Geometry: see drawing. Coordinates: mm, zero at the bounding-box minimum. Coordinates: 2 decimals unless noted, no trailing zeros. Write each loop counter-clockwise with the first axis right and the second up, starting at its lowest first coordinate (ties: lowest second). Pieces come first, ordered by that corner, then holes.
1) Line query: L1, parallel to Y at x = 280, z = 3.4. Output: solid intervals per line, ascending.
2) Section query B-B (y = 10). State how many separate pieces and enclosed holes the cut face has, then the cut area to 4 significant figures.
3) Section query A-A (x = 20). Output: boundary loops of the cut face in (y, z).
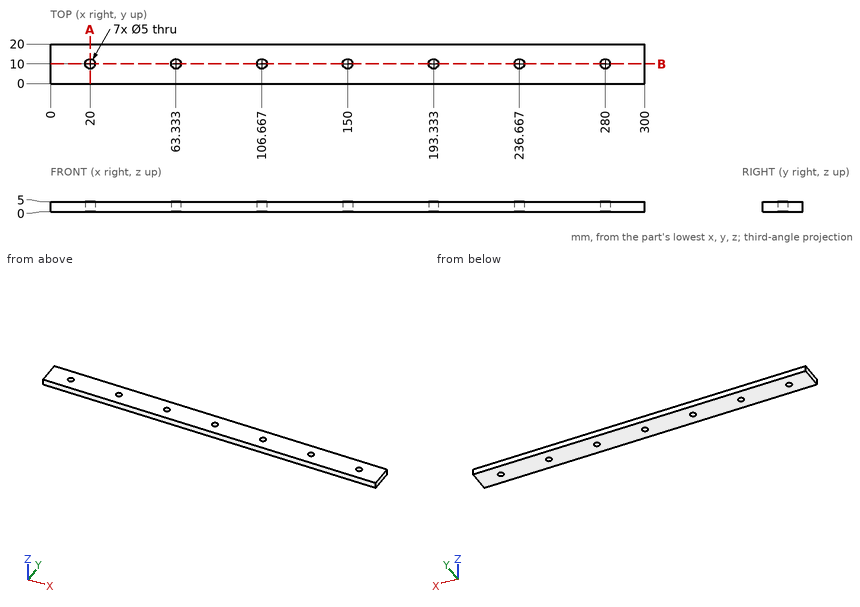
Answer:
1. L1: y = 0 to 7.5, 12.5 to 20
2. separate pieces: 8
2. enclosed holes: 0
2. area: 1,325 mm2
3. outline: (0, 0) - (7.5, 0) - (7.5, 5) - (0, 5) - close; (12.5, 0) - (20, 0) - (20, 5) - (12.5, 5) - close
